Source: CAD feature listing. Evaluate the final solid. Frame: model axes, mm. A direction names the side the tool comes from. Round coordinates to 2 decimals unless told otherwise and drop trailing zeros. Write each loop counter-clockwise with the first axis right and the second up, starting at its lowest first coordinate (ties: lowest second). Pieces come first, ordered by that corner, then holes. Notation, with made-up numbers: M -36,9.25 L -18,9.25 A19 cw -18,20.25 Z; hole C 60.5,47.25 d5. An arc over 180 degrees is marked long. Use a Markdown table: item, result.
```python
from build123d import *

# Parameters (mm, degrees)
BOSS_EXTRUDE1_DEPTH = 5
SKETCH1_3_W         = 4.8
SKETCH1_3_H         = 11.17
BOSS_EXTRUDE2_DEPTH = 3


with BuildPart() as part:
    # Sketch1 → Boss-Extrude1 (new body)
    with BuildSketch(Plane(origin=(0, 0, 0), x_dir=(1, 0, 0), z_dir=(0, 1, 0))):
        with BuildLine():
            ThreePointArc((-1.655620155, -5.519728682), (-2.405620155, -4.769728682), (-3.155620155, -5.519728682))
            Line((-3.155620155, -5.519728682), (-1.655620155, -5.519728682))
        make_face()
        with BuildLine():
            Line((-1.655620155, -5.519728682), (-3.155620155, -5.519728682))
            ThreePointArc((-3.155620155, -5.519728682), (-2.405620155, -6.269728682), (-1.655620155, -5.519728682))
        make_face()
    extrude(amount=BOSS_EXTRUDE1_DEPTH)

    # Sketch1_3 → Boss-Extrude2 (add)
    with BuildSketch(Plane(origin=(0, 0, 0), x_dir=(1, 0, 0), z_dir=(0, 1, 0))):
        Polygon((-4.805620155, -5.519728682), (-4.805620155, -3.119728682), (-15.975620155, -3.119728682), (-15.975620155, -7.919728682), (-4.805620155, -7.919728682), align=None)
        with BuildLine():
            Line((-0.005620155, -3.119728682), (-4.805620155, -3.119728682))
            Line((-4.805620155, -3.119728682), (-4.805620155, -5.519728682))
            Line((-4.805620155, -5.519728682), (-3.155620155, -5.519728682))
            ThreePointArc((-3.155620155, -5.519728682), (-2.405620155, -4.769728682), (-1.655620155, -5.519728682))
            Line((-1.655620155, -5.519728682), (-0.005620155, -5.519728682))
            Line((-0.005620155, -5.519728682), (-0.005620155, -3.119728682))
        make_face()
        with BuildLine():
            Line((-3.155620155, -5.519728682), (-4.805620155, -5.519728682))
            Line((-4.805620155, -5.519728682), (-4.805620155, -7.919728682))
            Line((-4.805620155, -7.919728682), (-0.005620155, -7.919728682))
            Line((-0.005620155, -7.919728682), (-0.005620155, -5.519728682))
            Line((-0.005620155, -5.519728682), (-1.655620155, -5.519728682))
            ThreePointArc((-1.655620155, -5.519728682), (-2.405620155, -6.269728682), (-3.155620155, -5.519728682))
        make_face()
        Polygon((11.164379845, -3.119728682), (-0.005620155, -3.119728682), (-0.005620155, -5.519728682), (-0.005620155, -7.919728682), (11.164379845, -7.919728682), align=None)
        with Locations((-2.405620155, -13.504728682)):
            Rectangle(SKETCH1_3_W, SKETCH1_3_H)
        with Locations((-2.405620155, 2.465271318)):
            Rectangle(SKETCH1_3_W, SKETCH1_3_H)
    extrude(amount=BOSS_EXTRUDE2_DEPTH)


solid = part.part
```
Q1. Section B-B on x = -10.5. Return loops of the section in (y, z).
Results are:
| item | result |
|---|---|
| outline | M 0,3.12 L 3,3.12 L 3,7.92 L 0,7.92 Z |
Q2. Section A-A on y = 1.1. Return loops of the section in (x, z).
Results are:
| item | result |
|---|---|
| outline | M -15.98,3.12 L -4.81,3.12 L -4.81,-8.05 L -0.01,-8.05 L -0.01,3.12 L 11.16,3.12 L 11.16,7.92 L -0.01,7.92 L -0.01,19.09 L -4.81,19.09 L -4.81,7.92 L -15.98,7.92 Z |
Q3. Reachability of faces 1 (the flat face through (-10, 1, 3.12)), 2 (the flat face through (6, 1, 7.92)), 3 (the cylindrical face through (-1.853, 3.986, 6.027)) from +Z, -Z, +X, -X, +Y, -Y: full face, straight path, thin tool, end or side. Return the list, or none.
Results are:
| item | result |
|---|---|
| face 1 | -Z, -X, +Y, -Y |
| face 2 | +Z, +X, +Y, -Y |
| face 3 | +Y |
Q4. Section C-C on z = 9.5. Return loops of the section in (x, y), plus the area to 3 significant figures.
Results are:
| item | result |
|---|---|
| outline | M -4.81,0 L -0.01,0 L -0.01,3 L -4.81,3 Z |
| area | 14.4 mm^2 |
Q5. Section D-D on y = 3.7. Return loops of the section in (x, z), plus the area to 3 significant figures.
Results are:
| item | result |
|---|---|
| outline | C -2.41,5.52 d1.5 |
| area | 1.77 mm^2 |
Q6. First-contact query: pin 1 Ø1.5 at (y, z) = (2, -3.5) entering from +X; pin 2 Ø1.5 at (x, y) = (8, 2) entering from +Z; pin 3 Ø1.5 at (y, z) = (1, -4) entering from -X. Flat tips, straight axial feed; report the tip coordinate or a pass-through.
Results are:
| item | result |
|---|---|
| pin 1 | x = -0.01 |
| pin 2 | z = 7.92 |
| pin 3 | x = -4.81 |
Q7. Line query: L1, parallel to Z at x = -11.25, y = 0.5; L2, parallel to Y at x = 7.25, z = 7.5; L3, parallel to X at y = 0.2, z = -0.5. Output: solid intervals per line, ascending.
Results are:
| item | result |
|---|---|
| L1 | 3.12 to 7.92 |
| L2 | 0 to 3 |
| L3 | -4.81 to -0.01 |
